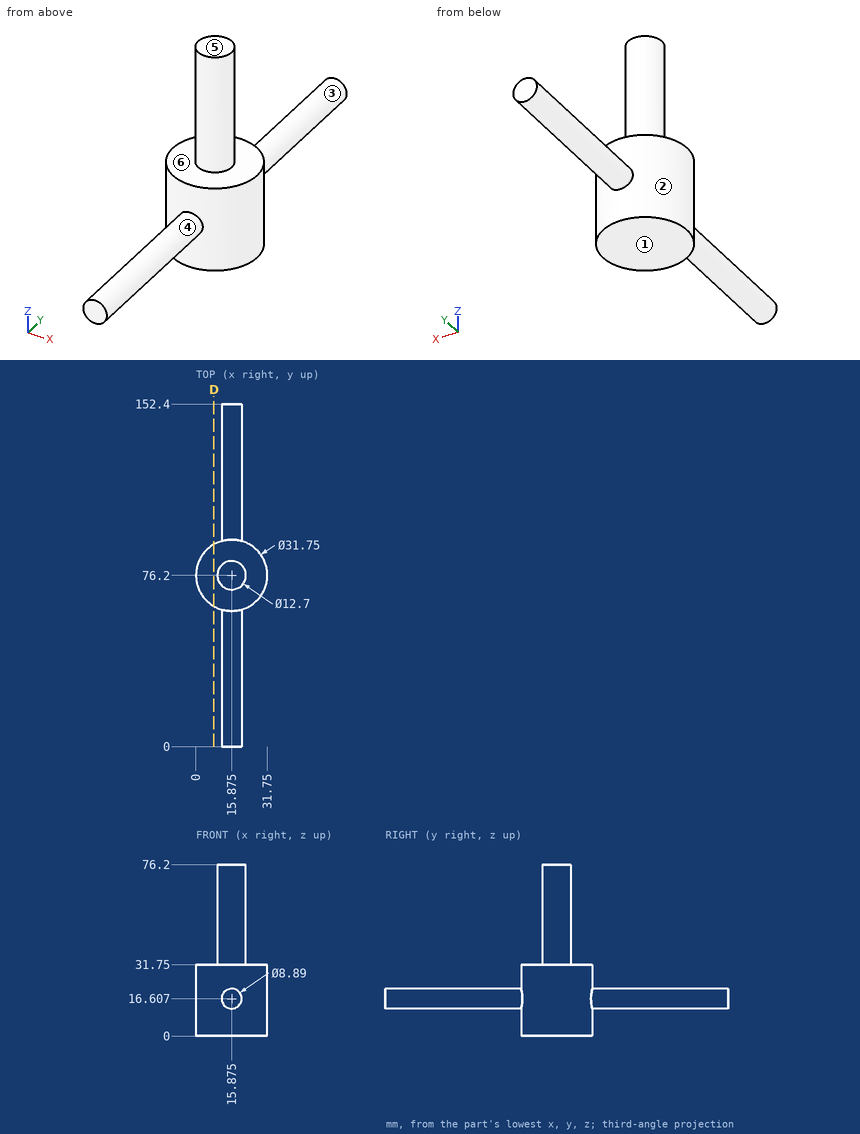
Design review of the part shown in the three views and the two pictorial views. Dimensions are in mm from the part's minimum x, y and z. A direction names the side the tool comes from. Round coordinates to 2 decimals unless told otherwise and drop trailing zeros. Order: outer loops, then holes, each group sorted by start corner. A loop starts at its lowest first (then second) coordinate and runs counter-clockwise, first axis right, second up.
Item 1: Draft analysis for pull direction X (two halves, no side actions). For the marked faces 1 and 2, state which applies: released by +X, released by -X, zero draft, split by the parting line, or undercut.
Working result:
face 1: zero draft
face 2: split by the parting line
Item 2: Add section D-D, the plane x = 8. State the section outline as (y, z) points.
Working result:
outline: (62.42, 0) - (89.98, 0) - (89.98, 31.75) - (62.42, 31.75) - close
Item 3: For pin 1 (1 mm diameter, centred on x = 13.5, y = 110.5, fed in from -Z); pin 2 (1 mm diameter, centred on y = 99.5, z = 18, fed in from -X); pin 3 (1.5 mm diameter, centred on y = 84.5, z = 39.5, fed in from -X); pin 4 (16 mm diameter, centred on x = 20, y = 70, fed in from +Z), all flat-tipped, find the tip position at first contact; note any pin that passes through.
Working result:
pin 1: stops at z = 12.58
pin 2: stops at x = 11.52
pin 3: passes through
pin 4: stops at z = 76.2
Item 4: To check wall thickness, follow probe 1 along Z at (x, y) = (27, 66); probe 2 along Z at (x, y) = (16, 25.5); probe 3 along Y at (x, z) = (2.5, 23.5). State the ranges of each line that lie inside material, in increasing order.
Working result:
probe 1: z = 0 to 31.75
probe 2: z = 12.16 to 21.05
probe 3: y = 67.65 to 84.75
Item 5: Machinability: for the marked faces 3, 4, 5 and 6, which of the approach directions +Z, -Z, +X, -X, +Y, -Y give a long, thin tool a straight path to every point of the face, cutting with its end or side? Answer none if there is none.
Working result:
face 3: +Y
face 4: -Y
face 5: +Z, +X, -X, +Y, -Y
face 6: +Z
